Model file for the job. Use its own axes, mm. Give positions to 0.01 mm unless a question says otherwise; leave off trailing zeros. Order: outer loops, then holes, each group sorted by start corner. A loop starts at its lowest first (then second) coordinate and runs counter-clockwise, first axis right, second up. Notation, with made-up numbers: M -39,-9 L 14,-9 A33 cw 14,30 Z; hole C 1.25,80.5 d8. An arc over 180 degrees is marked long. Return JSON: item names as keys, results as strings. Group by question number.
1. Wall check: probe 1 along X at (y, z) = (3.25, 12.7); probe 2 along X at (y, z) = (0, 8); probe 3 along Y at (x, z) = (-19.05, 11.75). Give the ranges that are in metal, low to high. Write a range as [from, to].
2. Slice it at C-C on y = 0. List the corners of the cut face in (x, z), then the cut area to 3 significant figures.
3. Two-plate mould, pull along Y, no slides. Class faces 1 (the face through (0, 6.35, 9)), 2 (the face through (-6.459, -0.089, 10.213)), 3 (the face through (17.086, 0.258, 9.392)): released by +Y, released by -Y, zero draft, split by the parting line, or undercut.
4. Slice it at B-B on z = 5.5. List the corners of the cut face in (x, y) (3 decimals), then the cut area to 3 significant figures.
5. Slice it at D-D on y = 2.5. List the corners of the cut face in (x, z), then the cut area to 3 significant figures.
6. Slice it at A-A on x = -6.35. List the corners of the cut face in (y, z).
Autodesk Inventor part; units mm, degrees
ref_plane "YZ Plane" through (0, 0, 0) normal (1, 0, 0) x (0, 1, 0)
ref_plane "XZ Plane" through (0, 0, 0) normal (0, 1, 0) x (-1, 0, 0)
ref_plane "XY Plane" through (0, 0, 0) normal (0, 0, 1) x (1, 0, 0)
sketch "Sketch1" plane through (0, 0, 0) normal (0, 0, 1) x (1, 0, 0)
  line L0 (25.4, -6.35) -> (-25.4, -6.35)
  line L1 (-25.4, -6.35) -> (-25.4, 6.35)
  line L2 (-25.4, 6.35) -> (25.4, 6.35)
  line L3 (25.4, 6.35) -> (25.4, -6.35)
  line L4 (25.4, -6.35) -> (-25.4, 6.35) construction
  line L5 (-25.4, -6.35) -> (25.4, 6.35) construction
  point P0 (0, 0)
  dimension "d0" = 50.8
  dimension "d1" = 12.7
extrude "Extrusion1" add sketch "Sketch1" along normal blind 19.05
sketch "Sketch2" plane through (-25.4, 6.35, 0) normal (0, 1, 0) x (1, 0, 0)
  line L0 (0, 0) -> (0, -19.05) construction
  line L1 (19.05, -12.7) -> (31.75, -12.7) construction
  line L2 (50.8, 0) -> (0, 0) construction
  line L3 (50.8, -19.05) -> (0, -19.05) construction
  point P0 (25.4, 0)
  point P1 (0, -9.525)
  point P2 (25.4, -12.7)
  point P3 (25.4, 0)
  point P4 (25.4, 0)
  dimension "d4" = 12.7
  dimension "d20" = 6.35
hole "Hole1" at (-6.35, 6.35, 12.7) at (6.35, 6.35, 12.7) direction (0, -1, 0) diameter 4.9784 end through all
sketch "Sketch3" plane through (0, 0, 19.05) normal (0, 0, 1) x (1, 0, 0)
  line L0 (-19.05, 0) -> (19.05, 0) construction
  line L1 (-25.4, 6.35) -> (-25.4, -6.35) construction
  line L2 (25.4, 6.35) -> (-25.4, 6.35) construction
  point P0 (0, 0)
  point P1 (-25.4, 0)
  point P2 (0, 0)
  point P3 (0, 6.35)
  dimension "d12" = 38.1
hole "Hole2" at (-19.05, 0, 19.05) at (19.05, 0, 19.05) direction (0, 0, -1) diameter 3.9624 end through all
fillet "Fillet1" radius 3.175 4 edges at (-25.4, 6.35, 9.525) (-25.4, -6.35, 9.525) (25.4, 6.35, 9.525) (25.4, -6.35, 9.525)
properties part number "CL7-014" material "Aluminum 6061"
Result:
{
 "1": {"probe 1": "x = [-25.4, -8.84], [-3.86, 3.86], [8.84, 25.4]", "probe 2": "x = [-25.4, -21.03], [-17.07, 17.07], [21.03, 25.4]", "probe 3": "y = [-6.35, -1.98], [1.98, 6.35]"},
 "2": {"outline": "M -25.4,0 L -21.03,0 L -21.03,19.05 L -25.4,19.05 Z; M -17.07,0 L 17.07,0 L 17.07,19.05 L -17.07,19.05 Z; M 21.03,0 L 25.4,0 L 25.4,19.05 L 21.03,19.05 Z; hole C -6.35,12.7 d4.98; hole C 6.35,12.7 d4.98", "area": "778 mm2"},
 "3": {"face 1": "released by +Y", "face 2": "zero draft", "face 3": "undercut"},
 "4": {"outline": "M -25.4,-3.175 A3.175 ccw -22.225,-6.35 L 22.225,-6.35 A3.175 ccw 25.4,-3.175 L 25.4,3.175 A3.175 ccw 22.225,6.35 L -22.225,6.35 A3.175 ccw -25.4,3.175 Z; hole C -19.05,0 d3.962; hole C 19.05,0 d3.962", "area": "612 mm2"},
 "5": {"outline": "M -25.4,0 L 25.4,0 L 25.4,19.05 L -25.4,19.05 Z; hole C -6.35,12.7 d4.98; hole C 6.35,12.7 d4.98", "area": "929 mm2"},
 "6": {"outline": "M -6.35,0 L 6.35,0 L 6.35,10.21 L -6.35,10.21 Z; M -6.35,15.19 L 6.35,15.19 L 6.35,19.05 L -6.35,19.05 Z"}
}
